Could you check a few things on this model? Use its own coordinates, in mm. Face numbers are marked on the shaded views. A direction names the side the tool comes from. Give positions to 0.01 mm unless a question says otherwise; leave off trailing zeros. Order: outer loops, then holes, each group sorted by start corner. A loop starts at its lowest first (then second) coordinate and runs counter-clockwise, first axis right, second up.
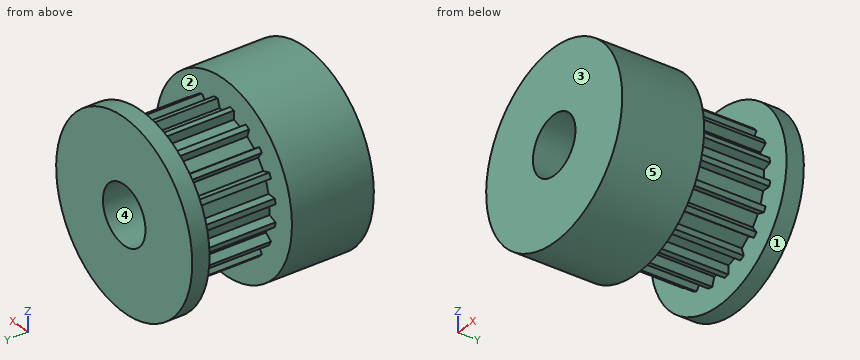
from build123d import *

# Parameters (mm, degrees)
SKETCH1_R           = 8
BOSS_EXTRUDE1_DEPTH = 7.1
SKETCH2_R           = 6.11
BOSS_EXTRUDE2_DEPTH = 7.14
SKETCH5_R           = 2.5
CUT_EXTRUDE2_DEPTH  = 16
CUT_EXTRUDE3_DEPTH  = 7.14
SKETCH8_R           = 8
BOSS_EXTRUDE4_DEPTH = 1.5
CUT_EXTRUDE4_START  = -15.74
SKETCH9_R           = 2.5
CUT_EXTRUDE4_DEPTH  = 15.74


with BuildPart() as part:
    # Sketch1 → Boss-Extrude1 (new body)
    with BuildSketch(Plane(origin=(0, 0, 0), x_dir=(1, 0, 0), z_dir=(0, 1, 0))):
        with Locations(Location((0, 0, 0), (0, 0, 270))):
            Circle(SKETCH1_R)
    extrude(amount=BOSS_EXTRUDE1_DEPTH)

    # Sketch2 → Boss-Extrude2 (add)
    with BuildSketch(Plane(origin=(0, 7.1, 0), x_dir=(1, 0, 0), z_dir=(0, 1, 0))):
        with Locations(Location((0, 0, 0), (0, 0, 270))):
            Circle(SKETCH2_R)
    extrude(amount=BOSS_EXTRUDE2_DEPTH)

    # Sketch5 → Cut-Extrude2 (cut)
    with BuildSketch(Plane.XZ):
        with Locations(Location((0, 0, 0), (0, 0, 270))):
            Circle(SKETCH5_R)
    extrude(amount=-CUT_EXTRUDE2_DEPTH, mode=Mode.SUBTRACT)

    # Sketch7 → Cut-Extrude3 (cut)
    with BuildSketch(Plane(origin=(0, 14.24, 0), x_dir=(1, 0, 0), z_dir=(0, 1, 0))):
        Polygon((-0.5, 5.36), (0.5, 5.36), (1, 6.86), (-1, 6.86), align=None)
        Polygon((3.070913098, 6.215230707), (2.131859348, 4.94315443), (1.180802832, 5.252171425), (1.168800065, 6.833264696), align=None)
        Polygon((4.841223825, 4.962071329), (3.555037449, 4.042438464), (2.746020455, 4.630223716), (3.223189836, 6.137641834), align=None)
        Polygon((6.137641834, 3.223189836), (4.630223716, 2.746020455), (4.042438464, 3.555037449), (4.962071329, 4.841223825), align=None)
        Polygon((6.833264696, 1.168800065), (5.252171425, 1.180802832), (4.94315443, 2.131859348), (6.215230707, 3.070913098), align=None)
        Polygon((6.86, -1), (5.36, -0.5), (5.36, 0.5), (6.86, 1), align=None)
        Polygon((6.215230707, -3.070913098), (4.94315443, -2.131859348), (5.252171425, -1.180802832), (6.833264696, -1.168800065), align=None)
        Polygon((4.962071329, -4.841223825), (4.042438464, -3.555037449), (4.630223716, -2.746020455), (6.137641834, -3.223189836), align=None)
        Polygon((3.223189836, -6.137641834), (2.746020455, -4.630223716), (3.555037449, -4.042438464), (4.841223825, -4.962071329), align=None)
        Polygon((1.168800065, -6.833264696), (1.180802832, -5.252171425), (2.131859348, -4.94315443), (3.070913098, -6.215230707), align=None)
        Polygon((-1, -6.86), (-0.5, -5.36), (0.5, -5.36), (1, -6.86), align=None)
        Polygon((-3.070913098, -6.215230707), (-2.131859348, -4.94315443), (-1.180802832, -5.252171425), (-1.168800065, -6.833264696), align=None)
        Polygon((-4.841223825, -4.962071329), (-3.555037449, -4.042438464), (-2.746020455, -4.630223716), (-3.223189836, -6.137641834), align=None)
        Polygon((-6.137641834, -3.223189836), (-4.630223716, -2.746020455), (-4.042438464, -3.555037449), (-4.962071329, -4.841223825), align=None)
        Polygon((-6.833264696, -1.168800065), (-5.252171425, -1.180802832), (-4.94315443, -2.131859348), (-6.215230707, -3.070913098), align=None)
        Polygon((-6.86, 1), (-5.36, 0.5), (-5.36, -0.5), (-6.86, -1), align=None)
        Polygon((-6.215230707, 3.070913098), (-4.94315443, 2.131859348), (-5.252171425, 1.180802832), (-6.833264696, 1.168800065), align=None)
        Polygon((-4.962071329, 4.841223825), (-4.042438464, 3.555037449), (-4.630223716, 2.746020455), (-6.137641834, 3.223189836), align=None)
        Polygon((-3.223189836, 6.137641834), (-2.746020455, 4.630223716), (-3.555037449, 4.042438464), (-4.841223825, 4.962071329), align=None)
        Polygon((-1.168800065, 6.833264696), (-1.180802832, 5.252171425), (-2.131859348, 4.94315443), (-3.070913098, 6.215230707), align=None)
    extrude(amount=-CUT_EXTRUDE3_DEPTH, mode=Mode.SUBTRACT)

    # Sketch8 → Boss-Extrude4 (add)
    with BuildSketch(Plane(origin=(0, 14.24, 0), x_dir=(1, 0, 0), z_dir=(0, 1, 0))):
        with Locations(Location((0, 0, 0), (0, 0, 270))):
            Circle(SKETCH8_R)
    extrude(amount=BOSS_EXTRUDE4_DEPTH)

    # Sketch9 → Cut-Extrude4 (cut)
    with BuildSketch(Plane(origin=(0, 15.74, 0), x_dir=(1, 0, 0), z_dir=(0, 1, 0)).offset(CUT_EXTRUDE4_START)):
        with Locations(Location((0, 0, 0), (0, 0, 90))):
            Circle(SKETCH9_R)
    extrude(amount=CUT_EXTRUDE4_DEPTH, mode=Mode.SUBTRACT)


solid = part.part
Item 1: Imagine slicing it at C-C on y = 3. List the corners of the cut face in (x, z) for me, then the cut area to 3 significant figures.
Findings:
outline: circle Ø16 at (0, 0); hole circle Ø5 at (0, 0)
area: 181 mm2
Item 2: Please list where these lines run through material, in increasing order: line 1 along X through (y, z) = (5.25, 0); line 2 along Y through (x, z) = (-6, 3); line 3 along Z through (x, y) = (0, 12.5).
Findings:
line 1: x = -8 to -2.5, 2.5 to 8
line 2: y = 0 to 7.1, 14.24 to 15.74
line 3: z = -5.36 to -2.5, 2.5 to 5.36
Item 3: We'd pull the mould along X, two halves only. Please class the marked faces 3, 4 and 5: +X half, -X half, draft (parallel to the pull), parting line (faces both ways), or undercut.
Findings:
face 3: draft
face 4: undercut
face 5: parting line
Item 4: Imagine slicing it at D-D on z = 7. List the corners of the cut face in (x, y) for me, then the cut area to 3 significant figures.
Findings:
outline: (-3.87, 0) - (3.87, 0) - (3.87, 7.1) - (-3.87, 7.1) - close; (-3.87, 14.24) - (3.87, 14.24) - (3.87, 15.74) - (-3.87, 15.74) - close
area: 66.6 mm2
Item 5: For the marked faces 1 and 2, which set-ups out of +Z, -Z, +X, -X, +Y, -Y let a thin tool reach every point of the face, with its end or its side?
Findings:
face 1: +Y, -Y
face 2: none
Item 6: For pin 1 (1 mm diameter, centred on y = 9, z = -1, fed in from +X); pin 2 (3 mm diameter, centred on x = -5.5, y = 7, fed in from -Z); pin 3 (5 mm diameter, centred on x = 6, y = 10, fed in from +Z), each with a flat end and sliding along its axis, tell me the tip position at first contact or that it passes through.
Findings:
pin 1: stops at x = 6.07
pin 2: stops at z = -6.93
pin 3: stops at z = 4.48
Item 7: Imagine slicing it at B-B on x = 0. List the corners of the cut face in (y, z) for me, then the cut area to 3 significant figures.
Findings:
outline: (0, -8) - (7.1, -8) - (7.1, -5.36) - (14.24, -5.36) - (14.24, -8) - (15.74, -8) - (15.74, -2.5) - (0, -2.5) - close; (0, 2.5) - (15.74, 2.5) - (15.74, 8) - (14.24, 8) - (14.24, 5.36) - (7.1, 5.36) - (7.1, 8) - (0, 8) - close
area: 135 mm2
Item 8: Imagine slicing it at A-A on z = 0. List the corners of the cut face in (x, y) for me, then the cut area to 3 significant figures.
Findings:
outline: (-8, 0) - (-2.5, 0) - (-2.5, 15.74) - (-8, 15.74) - (-8, 14.24) - (-5.36, 14.24) - (-5.36, 7.1) - (-8, 7.1) - close; (2.5, 0) - (8, 0) - (8, 7.1) - (5.36, 7.1) - (5.36, 14.24) - (8, 14.24) - (8, 15.74) - (2.5, 15.74) - close
area: 135 mm2
